Check sheet for the modelled part. Datum: model origin and axes. Units: mm. A direction names the side the tool comes from. Round coordinates to 2 decimals unless told otherwise and drop trailing zeros. Order: outer loops, then holes, each group sorted by start corner. A loop starts at its lowest first (then second) coordinate and runs counter-clockwise, first axis right, second up.
```python
from build123d import *

# Parameters (mm, degrees)
F3_SIZE   = 1
F6_DEPTH  = 19
F8_D      = 2.5
F8_DEPTH  = 14.2
F8_TIP    = 0.7510757738
F10_D     = 2
F10_DEPTH = 6
F10_TIP   = 0.600860619


# Not quite as in the source:
# - a fillet or chamfer that OpenCascade refuses, or shapes differently, is made with other operations: its cross-section is extruded or revolved along the edge and cut away or added


with BuildPart() as f2:
    # F0 (on Front) → F2 (revolve)
    with BuildSketch(Plane.XZ):
        Polygon((0, 10), (0, 0), (19, 0), (19, 19), (17.5, 19), (15.4792740578, 15.5), (13.5207259422, 15.5), (11.5, 19), (10, 19), (10, 10), align=None)
    revolve(axis=Axis((9.5, 0, 0), (-1, 0, 0)))

    # F3
    f3_edges = [f2.edges().sort_by_distance(p)[0] for p in [
        (0, 0, -10),
    ]]
    chamfer(f3_edges, length=F3_SIZE)

    # F4: chamfer of 0.25 on 10 edges, made by hand

    # F4_s1 → F4_t2 (revolve)
    with BuildSketch(Plane.XZ):
        Polygon((9.75, 10), (10, 10.25), (10, 10), align=None)
    revolve(axis=Axis((10, 0, 0), (-1, 0, 0)))

    # F4_s3 → F4_t4 (revolve)
    with BuildSketch(Plane.XZ):
        Polygon((15.3349364905, 15.5), (15.5514428415, 15.625), (15.4792740578, 15.5), align=None)
    revolve(axis=Axis((15.4792740578, 0, 0), (-1, 0, 0)))

    # F4_s5 → F4_t6 (revolve)
    with BuildSketch(Plane.XZ):
        Polygon((13.4485571585, 15.625), (13.6650635095, 15.5), (13.5207259422, 15.5), align=None)
    revolve(axis=Axis((13.5207259422, 0, 0), (-1, 0, 0)))

    # F4_s7 → F4_t8 (revolve, cut)
    with BuildSketch(Plane.XZ):
        Polygon((11.3556624327, 19), (11.5721687836, 18.875), (11.5, 19), align=None)
    revolve(axis=Axis((11.5, 0, 0), (-1, 0, 0)), mode=Mode.SUBTRACT)

    # F4_s9 → F4_t10 (revolve, cut)
    with BuildSketch(Plane.XZ):
        Polygon((10, 18.75), (10.25, 19), (10, 19), align=None)
    revolve(axis=Axis((10, 0, 0), (-1, 0, 0)), mode=Mode.SUBTRACT)

    # F4_s11 → F4_t12 (revolve, cut)
    with BuildSketch(Plane.XZ):
        Polygon((18.75, 19), (19, 18.75), (19, 19), align=None)
    revolve(axis=Axis((19, 0, 0), (-1, 0, 0)), mode=Mode.SUBTRACT)

    # F4_s13 → F4_t14 (revolve, cut)
    with BuildSketch(Plane.XZ):
        Polygon((17.4278312164, 18.875), (17.6443375673, 19), (17.5, 19), align=None)
    revolve(axis=Axis((17.5, 0, 0), (-1, 0, 0)), mode=Mode.SUBTRACT)

    # F5 (on Right) → F6 (cut, through all)
    with BuildSketch(Plane.YZ):
        with BuildLine():
            Line((-6.4, -1.5), (-4.7696960071, -1.5))
            ThreePointArc((-4.7696960071, -1.5), (5, 0), (-4.7696960071, 1.5))
            Line((-4.7696960071, 1.5), (-6.4, 1.5))
            Line((-6.4, 1.5), (-6.4, -1.5))
        make_face()
    extrude(amount=F6_DEPTH, mode=Mode.SUBTRACT)

    # F8
    with Locations(Plane.XZ.offset(10)):
        with Locations((5, 0)):
            Hole(F8_D / 2, depth=F8_DEPTH)
            with Locations((0, 0, -(F8_DEPTH + F8_TIP / 2))):  # 118° drill point
                Cone(0, F8_D / 2, F8_TIP, mode=Mode.SUBTRACT)

    # F10
    with Locations(Plane.YZ.offset(19)):
        with Locations((0, 8.75), (0, -8.75)):
            Hole(F10_D / 2, depth=F10_DEPTH)
            with Locations((0, 0, -(F10_DEPTH + F10_TIP / 2))):  # 118° drill point
                Cone(0, F10_D / 2, F10_TIP, mode=Mode.SUBTRACT)


solid = f2.part
```
Item 1: Sectioned sample at B-B (z = 0). State how many separate pieces and enclosed holes the cut face has, and give its area (3 significant figures).
Answer:
separate pieces: 3
enclosed holes: 0
area: 287 mm2
Item 2: Sectioned sample at A-A (x = 8.5). Record the cut outline in (y, z).
Answer:
outline: circle Ø20 at (0, 0); hole (-6.4, -1.5) - (-4.77, -1.5) arc R5 ccw (long way) to (-4.77, 1.5) - (-6.4, 1.5) - close
Item 3: Scan lines: line 1 along X through (y, z) = (-5, -13.5); line 2 along Y through (x, z) = (17.7, -8.75); line 3 along X through (y, z) = (14, -8). Record each from-to range of solid material in increasing order.
Answer:
line 1: x = 10 to 19
line 2: y = -16.87 to -1, 1 to 16.87
line 3: x = 10 to 13.16, 15.84 to 19
Item 4: Go/stop test with flat-tipped pins: P1, Ø2, axis at x = 5.5, z = -8.5, coming from the -Y side; P2, Ø1, axis at y = -2.5, z = 1, coming from the -X side; P3, Ø3, axis at x = 5, z = 0, coming from the -Y side; P4, Ø4, axis at x = 14.5, z = 9.5, coming from the +Y side. Record where each tip stops, or that it passes through.
Answer:
P1: stops at y = -6.61
P2: passes through
P3: stops at y = -10
P4: stops at y = 14.61
Item 5: Release check for a two-part mould opening along Z. For faces 1 (the cylindrical face through (10.795, -16.856, 8.767)), 2 (the flat face through (9, -6, 1.5)), 3 (the flat face through (0, -4, 4)) record: released by +Z, released by -Z, zero draft, split by the parting line, or undercut.
Answer:
face 1: split by the parting line
face 2: undercut
face 3: zero draft
Item 6: Access from +Z, -Z, +X, -X, +Y, -Y to the whole of each face (thin tool, end or side, straight path). Record for faces 4 (the conical face through (15.643, 15.648, -2.055)), 5 (the cylindrical face through (15.96, 0.13, -7.76)), 6 (the cylindrical face through (5.31, -9.76, -2.17)), 7 (the flat face through (9, -6.4, 0)).
Answer:
face 4: none
face 5: +X
face 6: -X
face 7: +X, -X
Item 7: Sectioned sample at C-C (x = 5). Record the cut outline in (y, z), and give its area (3 significant figures).
Answer:
outline: (-9.92, -1.25) arc R10 ccw (long way) to (-9.92, 1.25) - (-6.4, 1.25) - (-6.4, 1.5) - (-4.77, 1.5) arc R5 cw (long way) to (-4.77, -1.5) - (-6.4, -1.5) - (-6.4, -1.25) - close
area: 222 mm2
